Drawing for the job (mm, zero at the part's lowest x, y, z). Give positions to 0.01 mm unless a question says otherwise; leave off trailing zeros. Loops run counter-clockwise (first coordinate to the right, second up) from the corner with the lowest first, then second, coordinate; pieces in that order, holes last. Notation, with made-up numbers: (-2, 85) -> (7, 85) arc R22 ccw to (7, 107) -> close; hole circle Ø10 at (-22, 81.25). An arc over 180 degrees is marked (long way). Use CSV: the item, a comma, the result in double quotes. Start each with the question number.
(1) Cut at A-A on y = 36.5. Write the cut outline in (x, z).
(2) Drill centre lines: probe 1 along X at (y, z) = (39.5, 22) (1 decimal); probe 2 along X at (y, z) = (46.5, 10.5); probe 3 along Y at (x, z) = (31.5, 12). Where is each one in solid material? Low to high.
(3) Pull direction X, two halves, no side cores. Call the marked faces 1, 2, 3 and 4: pulls with the +X half, pulls with the -X half, needs draft (parallel to the pull), parting line crosses it, or undercut.
(4) Cut at C-C on z = 22. Write the cut outline in (x, y) (1 decimal), then the cut area to 3 significant figures.
(5) Cut at B-B on x = 33. Write the cut outline in (y, z) (1 decimal).
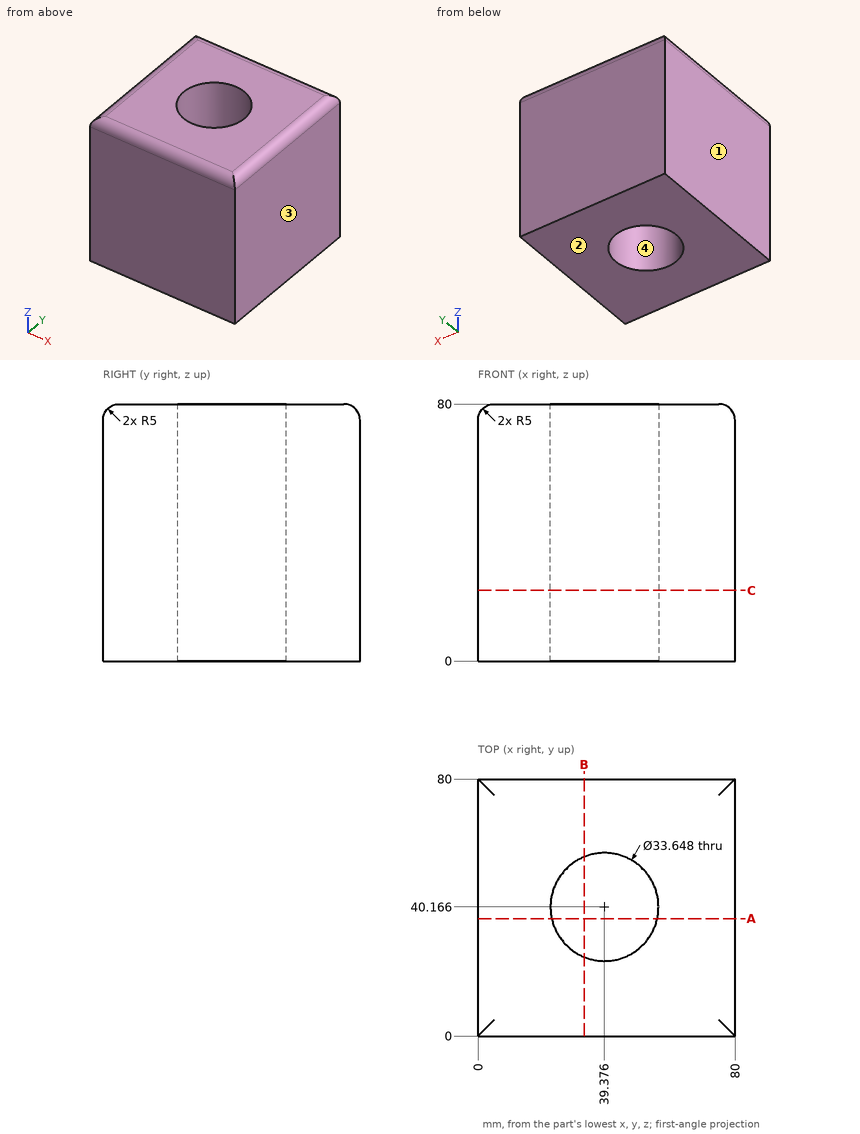
Check result:
1,outline,"(0, 0) -> (22.96, 0) -> (22.96, 80) -> (5, 80) arc R5 ccw to (0, 75) -> close; (55.8, 0) -> (80, 0) -> (80, 75) arc R5 ccw to (75, 80) -> (55.8, 80) -> close"
2,probe 1,"0 to 22.6, 56.2 to 80"
2,probe 2,"0 to 23.79, 54.96 to 80"
2,probe 3,"0 to 25.3, 55.03 to 80"
3,face 1,"pulls with the -X half"
3,face 2,"needs draft"
3,face 3,"pulls with the +X half"
3,face 4,"undercut"
4,outline,"(0, 0) -> (80, 0) -> (80, 80) -> (0, 80) -> close; hole circle Ø33.6 at (39.4, 40.2)"
4,area,"5,510 mm²"
5,outline,"(0, 0) -> (24.6, 0) -> (24.6, 80) -> (5, 80) arc R5 ccw to (0, 75) -> close; (55.7, 0) -> (80, 0) -> (80, 75) arc R5 ccw to (75, 80) -> (55.7, 80) -> close"
